Autodesk Inventor part; units mm, degrees
ref_plane "YZ Plane" through (0, 0, 0) normal (1, 0, 0) x (0, 1, 0)
ref_plane "XZ Plane" through (0, 0, 0) normal (0, 1, 0) x (-1, 0, 0)
sketch "Skizze1" plane through (0, 0, 0) normal (0, 0, 1) x (1, 0, 0)
  line L0 (-16, 20) -> (16, 20)
  line L1 (16, 20) -> (16, -20)
  line L2 (16, -20) -> (-16, -20)
  line L3 (-16, -20) -> (-16, 20)
  line L4 (-16, 20) -> (16, -20) construction
  line L5 (16, 20) -> (-16, -20) construction
  point P0 (0, 0)
  dimension "d0" = 32
  dimension "d1" = 40
extrude "Extrusion1" add sketch "Skizze1" along normal blind 15
sketch "Skizze2" plane through (-16, -20, 0) normal (0, -1, 0) x (1, 0, 0)
  line L0 (0, 15) -> (32, 15)
  line L1 (0, 0) -> (0, 15)
  line L2 (32, 0) -> (0, 0)
  line L3 (32, 0) -> (32, 15)
  line L4 (32, 15) -> (0, 15)
  circle A0 centre (16, 15) radius 10
  point P0 (16, 0)
  dimension "d4" = 20
extrude "Extrusion2" cut sketch "Skizze2" against normal blind 15 contours A0 L0 | L0 A0
sketch "Skizze3" plane through (-16, -5, 0) normal (0, -1, 0) x (1, 0, 0)
  line L0 (0, 0) -> (0, 15)
  line L1 (32, 0) -> (0, 0)
  line L2 (32, 0) -> (32, 15)
  line L3 (26, 15) -> (32, 15)
  line L4 (0, 15) -> (6, 15)
  line L5 (6, 15) -> (26, 15)
  circle A0 centre (16, 15) radius 10.5
  point P0 (16, 0)
  dimension "d7" = 21
extrude "Extrusion3" cut sketch "Skizze3" against normal blind 5 contours A0 L3 L5 L4 | L4 L5 L3 A0
sketch "Skizze4" plane through (-16, 0, 0) normal (0, -1, 0) x (1, 0, 0)
  line L0 (5.5, 15) -> (26.5, 15)
  circle A0 centre (16, 15) radius 12.5
  point P0 (16, 0)
  dimension "d10" = 25
extrude "Extrusion4" cut sketch "Skizze4" against normal through all
sketch "Skizze5" plane through (0, 0, 15) normal (0, 0, 1) x (1, 0, 0)
  line L0 (-16, 20) -> (-16, -20)
  line L1 (-16, -20) -> (-10, -20)
  line L2 (-10, -20) -> (-10, -5)
  line L3 (10, -5) -> (10, -20)
  line L4 (10, -20) -> (16, -20)
  line L5 (16, -20) -> (16, 20)
  circle A0 centre (-13, -13) radius 1.8
  circle A1 centre (13, -13) radius 1.8
  point P0 (0, 0)
  dimension "d13" = 3.6
  dimension "d14" = 3.6
  dimension "d15" = 7
  dimension "d16" = 7
  dimension "d17" = 3
  dimension "d18" = 3
extrude "Extrusion5" cut sketch "Skizze5" against normal through all
sketch "Skizze6" plane through (0, 0, 0) normal (0, 0, 1) x (1, 0, 0)
  line L0 (16, 20) -> (16, -20)
  line L1 (-16, 20) -> (16, 20)
  line L2 (16, 20) -> (16, 10.5)
  line L3 (16, 10.5) -> (-16, 10.5)
  line L4 (-16, 10.5) -> (-16, 20)
  point P0 (0, 0)
  dimension "d21" = 9.5
extrude "Extrusion6" cut sketch "Skizze6" along normal blind 15
properties part number "5 Objektivhalterung oben 29112018"
Geometry: final body of the model. Coordinates: model frame, mm. A direction names the side the tool comes from. Coordinates: 2 decimals unless noted, no trailing zeros. Order: outer loops, then holes, each group sorted by start corner. A loop starts at its lowest first (then second) coordinate and runs counter-clockwise, first axis right, second up. Notation, with made-up numbers: (36, 32) - (86, 32) arc R16 cw to (86, 51) - close; hole circle Ø2 at (9, 2.25). An arc over 180 degrees is marked (long way). Write each question's results on one line, items separated by ' | '.
1) Pull-direction query (X, two-part tool) for faces 3 (the flat face through (-16, -5, 7)), 4 (the flat face through (-2, -5, 5)), 5 (the flat face through (0, -20, 4)); classes: pulls with the +X half, pulls with the -X half, needs draft (parallel to the pull), parting line crosses it, or undercut.
Results list:
face 3: pulls with the -X half | face 4: undercut | face 5: needs draft
2) Section B-B, the plane y = -14. Return loops of the section in (x, z), plus the area to 3 significant figures.
Results list:
outline: (-16, 0) - (-14.5, 0) - (-14.5, 15) - (-16, 15) - close; (-11.5, 0) - (11.5, 0) - (11.5, 15) - (10, 15) arc R10 cw to (-10, 15) - (-11.5, 15) - close; (14.5, 0) - (16, 0) - (16, 15) - (14.5, 15) - close | area: 233 mm^2
3) Section D-D, the plane y = -1. Return loops of the section in (x, z).
Results list:
outline: (-16, 0) - (16, 0) - (16, 15) - (10.5, 15) arc R10.5 cw to (-10.5, 15) - (-16, 15) - close
4) Set-up query: faces 1 (the cylindrical face through (-0.275, 5.176, 2.503)), 2 (the cylindrical face through (0, -13, 5)). Return all of +Z, -Z, +X, -X, +Y, -Y with unobstructed straight access to the full face (end or side cutting, diameter ignored); none if empty.
Results list:
face 1: +Z, +Y | face 2: +Z, +Y, -Y
5) Pin query (flat end, axial travel): pin 1 (6.5 mm diameter, centred on x = -6, z = 8, fed in from +Y); pin 2 (12 mm diameter, centred on x = -4, y = 6, fed in from +Z); pin 3 (2 mm diameter, centred on x = 13, y = -13, fed in from -Z); pin 4 (1.5 mm diameter, centred on x = -3, y = -11.5, fed in from +Z). Return the tip coordinate at first contact, or that it passes through.
Results list:
pin 1: y = 0 | pin 2: z = 7.5 | pin 3: through | pin 4: z = 5.73
6) Section C-C, the plane x = -13. Return loops of the section in (y, z), plus the area to 4 significant figures.
Results list:
outline: (-20, 0) - (-14.8, 0) - (-14.8, 15) - (-20, 15) - close; (-11.2, 0) - (10.5, 0) - (10.5, 15) - (-11.2, 15) - close | area: 403.5 mm^2
7) Section A-A, the plane z = 11. Return loops of the section in (x, y).
Results list:
outline: (-16, -20) - (-9.17, -20) - (-9.17, -5) - (-9.71, -5) - (-9.71, 0) - (-11.84, 0) - (-11.84, 10.5) - (-16, 10.5) - close; (9.17, -20) - (16, -20) - (16, 10.5) - (11.84, 10.5) - (11.84, 0) - (9.71, 0) - (9.71, -5) - (9.17, -5) - close; hole circle Ø3.6 at (-13, -13); hole circle Ø3.6 at (13, -13)
8) Line query: line 1 (Y direction, x = 13, z = 9.5); line 2 (X direction, y = -14, z = 13.5); line 3 (Y direction, x = -3, z = 3.5). Output: solid intervals per line, ascending. Write a range as from..to.
Results list:
line 1: -20..-14.8, -11.2..10.5 | line 2: -16..-14.5, -11.5..-9.89, 9.89..11.5, 14.5..16 | line 3: -20..0
